Part model, mm, in its own coordinate system. A direction names the side the tool comes from. Give positions to 0.01 mm unless a question says otherwise; leave off trailing zeros. Order: outer loops, then holes, each group sorted by start corner. A loop starts at its lowest first (then second) coordinate and runs counter-clockwise, first axis right, second up. Notation, with made-up numbers: M 76.5,39 L 92.5,39 A25 ccw 92.5,53 Z; hole C 37.5,77.25 d4. An arc over 180 degrees is marked long. Return JSON: item names as keys, results as strings.
from build123d import *

# Parameters (mm, degrees)
SKETCH1_R           = 12.7
BOSS_EXTRUDE1_DEPTH = 63.5
BOSS_EXTRUDE2_DEPTH = 50.8


with BuildPart() as part:
    # Sketch1 → Boss-Extrude1 (new body, symmetric)
    with BuildSketch(Plane(origin=(0, 0, 0), x_dir=(0, 0, -1), z_dir=(1, 0, 0))):
        Circle(SKETCH1_R)
    extrude(amount=BOSS_EXTRUDE1_DEPTH, both=True)

    # Sketch2 → Boss-Extrude2 (add)
    with BuildSketch(Plane(origin=(63.5, 0, 0), x_dir=(0, 0, -1), z_dir=(1, 0, 0))):
        with BuildLine():
            ThreePointArc((12.7, 0), (6.35, 10.998522628), (-6.35, 10.998522628))
            Line((-6.35, 10.998522628), (-6.35, -10.998522628))
            ThreePointArc((-6.35, -10.998522628), (6.35, -10.998522628), (12.7, 0))
        make_face()
    boss_extrude2 = extrude(amount=BOSS_EXTRUDE2_DEPTH)

    # Mirror1: Boss-Extrude2 across plane
    add(boss_extrude2.mirror(Plane(origin=(0, 0, 0), x_dir=(0, 0, 1), z_dir=(1, 0, 0))))


solid = part.part
Q1. Band-saw the part on A-A (y = -6.5). Give the cut face in (x, z), then the cut area to 3 significant figures.
Established:
{"outline": "M -114.3,-10.91 L 114.3,-10.91 L 114.3,6.35 L 63.5,6.35 L 63.5,10.91 L -63.5,10.91 L -63.5,6.35 L -114.3,6.35 Z", "area": "4,520 mm²"}
Q2. 3-axis set-ups, long thin cutter, end or side, ignore diameter. For faces 1 (the flat face through (-63.5, 0, 9)), 2 (the flat face through (63.5, 0, 9)), 3 (the flat face through (-114.3, 0, -1)): which of +Z, -Z, +X, -X, +Y, -Y reach the whole face in a straight line?
Established:
{"face 1": "+Z, -X, +Y, -Y", "face 2": "+Z, +X, +Y, -Y", "face 3": "+Z, -Z, -X, +Y, -Y"}
Q3. Probe line 1 along X through (y, z) = (4, 6.75); line 2 along Z through (x, y) = (103.5, -0.5); line 3 along Y through (x, z) = (-47, -5). List the from-to ranges inside material, lowest first.
Established:
{"line 1": "x = -63.5 to 63.5", "line 2": "z = -12.69 to 6.35", "line 3": "y = -11.67 to 11.67"}
Q4. Pin check, flat tips, straight feed: pin 1 (4 mm diameter, centred on x = 64.5, z = 4, fed in from +Y); pin 2 (1.5 mm diameter, centred on x = -1.5, z = -8.5, fed in from +Y); pin 3 (1.9 mm diameter, centred on y = 5, z = 10.5, fed in from +X). Stop position of each tip, or through.
Established:
{"pin 1": "stops at y = 12.54", "pin 2": "stops at y = 10.06", "pin 3": "stops at x = 63.5"}
Q5. Band-saw the part on D-D (x = -18). Give the cut face in (y, z), then the cut area to 3 significant figures.
Established:
{"outline": "C 0,0 d25.4", "area": "507 mm²"}
Q6. Band-saw the part on C-C (z = -10.5). Give the cut face in (x, y).
Established:
{"outline": "M -114.3,-7.14 L 114.3,-7.14 L 114.3,7.14 L -114.3,7.14 Z"}
Q7. Band-saw the part on B-B (x = 89). Give the cut face in (y, z), then the cut area to 3 significant figures.
Established:
{"outline": "M -11,6.35 A12.7 ccw long 11,6.35 Z", "area": "408 mm²"}
